Work out the finished part from the listing and answer in its coordinate system (mm). Coordinates: 2 decimals unless noted, no trailing zeros. Order: outer loops, then holes, each group sorted by start corner. A loop starts at its lowest first (then second) coordinate and runs counter-clockwise, first axis right, second up. Notation, with made-up numbers: M 81,59.5 L 106,59.5 A32 cw 106,93.5 Z; hole C -19.75,14.25 d8. An arc over 180 degrees is marked long. Use a Markdown table: item, result.
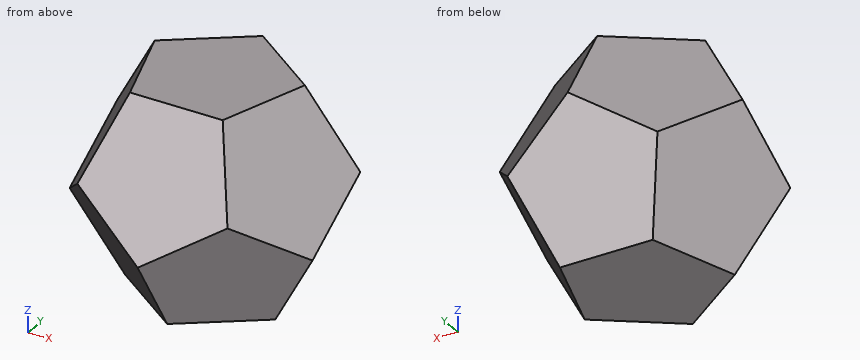
Solid Edge part; units mm, degrees
sketch "Sketch1" plane through (0, 0, 0) normal (1, 0, 0) x (0, 1, 0)
  line L0 (0, 125.7387) -> (0, -58.9278)
  arc A0 (0, 125.7388) -> (0, -58.9278) centre (0, 33.4055) cw
revolve "RevolvedProtrusion1" add sketch "Sketch1" angle 360 about axis through (0, 0, 125.7387) along (0, 0, -1)
sketch "Sketch2" plane through (0, 0, 0) normal (1, 0, 0) x (0, 1, 0)
  line L0 (-41.2915, 25.5195) -> (-25.5195, 0)
  line L1 (-20.6457, 66.811) -> (-41.2915, 25.5195)
  line L2 (25.5195, 66.811) -> (-20.6457, 66.811)
  line L3 (41.2915, 41.2915) -> (25.5195, 66.811)
  line L4 (20.6457, 0) -> (41.2915, 41.2915)
extrude "Cutout1" cut sketch "Sketch2" along normal mid plane 232.5761 material side at (0, -33.448, 12.7335)
pattern_circular "Pattern1" count 5 over 360 about axis through (0, 0, 66.811) along (0, 0, 1) of "Cutout1"
sketch "Sketch3" plane through (0, 0, 0) normal (0, 0, 1) x (1, 0, 0)
  line L0 (24.2705, -7.886) -> (15, 20.6457)
  line L1 (15, 20.6457) -> (-15, 20.6457)
  line L2 (-15, 20.6457) -> (-24.2705, -7.886)
  line L3 (-24.2705, -7.886) -> (0, -25.5195)
  line L4 (0, -25.5195) -> (24.2705, -7.886)
extrude "ExtrudedCutout_8" cut sketch "Sketch3" against normal blind 119.4
(1) A cutting plane is placed at B-B (y = -4). Determine the outline of the cut face in (x, z), then the cut area to 3 significant figures.
Conclusion:
| item | result |
|---|---|
| outline | M -39.27,30.93 L -23.01,0 L 23.01,0 L 39.27,30.93 L 20.41,66.81 L -20.41,66.81 Z |
| area | 4,070 mm2 |
(2) A cutting plane is placed at A-A (z = 30.5). Determine the outline of the cut face in (x, y).
Conclusion:
| item | result |
|---|---|
| outline | M -39.27,-4.7 L -34.53,-19.28 L -7.66,-38.8 L 7.66,-38.8 L 34.53,-19.28 L 39.27,-4.7 L 29.01,26.89 L 16.61,35.9 L -16.61,35.9 L -29.01,26.89 Z |
(3) A cutting plane is placed at C-C (x = 16.5). Determine the outline of the cut face in (y, z).
Conclusion:
| item | result |
|---|---|
| outline | M -35.93,36.24 L -13.53,0 L 16.03,0 L 22.71,4.13 L 35.93,30.57 L 13.53,66.81 L -16.03,66.81 L -22.71,62.68 Z |
(4) Straight lines are drawn through the part: L1, parallel to Z at x = -10, y = 22; L2, parallel to Y at x = 19, z = 52; L3, parallel to X at y = 6, z = 7. For each, find the intervals that lie inside material, in ascending order.
Conclusion:
| item | result |
|---|---|
| L1 | 2.71 to 60.75 |
| L2 | -28.05 to 20.87 |
| L3 | -23.44 to 23.44 |
(5) Given P1, Ø2, axis at x = -7, y = -25.5, coming from the -Z side; P2, Ø8, axis at x = -31, y = 14, coming from the +Z side; P3, Ø2, axis at x = 30.5, y = -5, coming from the +Z side, each flat-ended and moving along its own axis, determine where each tip first touches the part or whether it passes through.
Conclusion:
| item | result |
|---|---|
| P1 | z = 6.2 |
| P2 | z = 57.01 |
| P3 | z = 49 |
(6) A cutting plane is placed at D-D (z = 39). Determine the outline of the cut face in (x, y), then the cut area to 3 significant figures.
Conclusion:
| item | result |
|---|---|
| outline | M -39.27,9.05 L -26.45,-30.41 L -20.74,-34.55 L 20.74,-34.55 L 26.45,-30.41 L 39.27,9.05 L 37.09,15.76 L 3.53,40.15 L -3.53,40.15 L -37.09,15.76 Z |
| area | 4,290 mm2 |
